from build123d import *

# Parameters (mm, degrees)
F0_W      = 50
F0_H      = 50
F1_DEPTH  = 12
F3_DEPTH  = 12
F5_W      = 7.196964696
F5_H      = 12
F6_DEPTH  = 25
F7_W      = 5.4
F7_H      = 5.4
F8_DEPTH  = 25
F9_W      = 5.4
F9_H      = 5.4
F9_W_2    = 4.6
F9_H_2    = 4.6
F10_DEPTH = 1
F11_R     = 0.19999
F13_W     = 25
F13_H     = 12
F14_DEPTH = 50
F15_W     = 25
F15_H     = 12
F16_DEPTH = 25
F17_COUNT = 4


# Not quite as in the source:
# - a fillet or chamfer that OpenCascade refuses, or shapes differently, is made with other operations: its cross-section is extruded or revolved along the edge and cut away or added
# - a fillet or chamfer is up to 0.001 mm smaller than in the source, because OpenCascade refuses the exact size


with BuildPart() as f1:
    # F0 (on Top) → F1 (new body)
    with BuildSketch(Plane.XY):
        Rectangle(F0_W, F0_H)
    extrude(amount=F1_DEPTH)

    # F2 (on face) → F3 (join)
    with BuildSketch(Plane(origin=(-25, 0, 0), x_dir=(0, -1, 0), z_dir=(-1, 0, 0))):
        with BuildLine():
            ThreePointArc((0, 0), (4.2426406871, 1.7573593129), (6, 6))
            ThreePointArc((6, 6), (4.2426406871, 10.2426406871), (0, 12))
            ThreePointArc((0, 12), (-6, 6), (0, 0))
        make_face()
    extrude(amount=F3_DEPTH)

    # F4: fillet of radius 6 on 1 edges, made by hand

    # F4_s1 → F4_t2 (revolve, cut)
    with BuildSketch(Plane.XZ):
        with BuildLine():
            ThreePointArc((-31, 12), (-35.2426406871, 10.2426406871), (-37, 6))
            Line((-37, 6), (-37.12, 6))
            Line((-37.12, 6), (-37.12, 12.12))
            Line((-37.12, 12.12), (-31, 12.12))
            Line((-31, 12.12), (-31, 12))
        make_face()
    revolve(axis=Axis((-37, 0, 6), (1, 0, 0)), mode=Mode.SUBTRACT)

    # F5 (on face) → F6 (cut)
    with BuildSketch(Plane(origin=(-25, 0, 0), x_dir=(0, -1, 0), z_dir=(-1, 0, 0))):
        with Locations((3.598482348, 6)):
            Rectangle(F5_W, F5_H)
    extrude(amount=F6_DEPTH, mode=Mode.SUBTRACT)

    # F7 (on face) → F8 (cut)
    with BuildSketch(Plane.XZ):
        with Locations((-31, 6)):
            Rectangle(F7_W, F7_H)
    extrude(amount=-F8_DEPTH, mode=Mode.SUBTRACT)

    # F9 (on face) → F10 (join)
    with BuildSketch(Plane.XZ):
        with Locations((-31, 6)):
            Rectangle(F9_W, F9_H)
        with Locations((-31, 6)):
            Rectangle(F9_W_2, F9_H_2, mode=Mode.SUBTRACT)
    extrude(amount=-F10_DEPTH)

    # F11 (radius 0.2 in the source; OpenCascade refuses exactly that, so slightly less here)
    f11_edges = [f1.edges().sort_by_distance(p)[0] for p in [
        (-28.7, 1, 6),
        (-28.3, 1, 6),
        (-31, 1, 8.7),
        (-31, 1, 8.3),
        (-33.7, 1, 6),
        (-33.3, 1, 6),
        (-31, 1, 3.3),
        (-31, 1, 3.7),
    ]]
    fillet(f11_edges, radius=F11_R)

    # F13 (on face) → F14 (cut)
    with BuildSketch(Plane(origin=(-25, 0, 0), x_dir=(0, -1, 0), z_dir=(-1, 0, 0))):
        with Locations((12.5, 6)):
            Rectangle(F13_W, F13_H)
    extrude(amount=-F14_DEPTH, mode=Mode.SUBTRACT)

    # F15 (on face) → F16 (cut)
    with BuildSketch(Plane(origin=(0, 25, 0), x_dir=(-1, 0, 0), z_dir=(0, 1, 0))):
        with Locations((-12.5, 6)):
            Rectangle(F15_W, F15_H)
    extrude(amount=-F16_DEPTH, mode=Mode.SUBTRACT)

    # F17: F1 ×4 about axis
    f17_axis = Axis((0, 0, 13.6458836496), (0, 0, 1))


with BuildPart() as f1_1:
    add(f1.part)
    for i in range(1, F17_COUNT):
        add(f1.part.rotate(f17_axis, i * 360 / F17_COUNT))


solid = f1_1.part
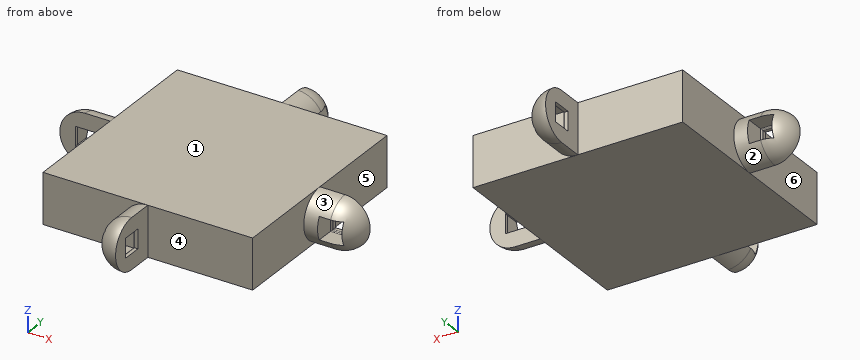
CAD build for the part. Positions are in the model's coordinates, mm. Face numbers are marked on the shaded views. A direction names the side the tool comes from. Give positions to 0.01 mm unless a question says otherwise; leave off trailing zeros. Order: outer loops, then holes, each group sorted by start corner. A loop starts at its lowest first (then second) coordinate and runs counter-clockwise, first axis right, second up. Notation, with made-up numbers: (-31.5, 66) - (-10.5, 66) arc R11 cw to (-10.5, 75) - close; hole circle Ø11 at (-11.75, 51.25). An arc over 180 degrees is marked (long way). Answer in a Markdown table with one row per item.
1. Saw through at D-D, the plane z = 1.75. Give the cut face in (x, y), plus the area to 3 significant figures.
Data:
| item | result |
|---|---|
| outline | (-35.24, 0) - (-25, 0) - (-25, -25) - (-4.24, -25) - (-4.24, -31) arc R4.24 ccw to (0, -35.24) - (0, -25) - (25, -25) - (25, -4.24) - (31, -4.24) arc R4.24 ccw to (35.24, 0) - (25, 0) - (25, 25) - (4.24, 25) - (4.24, 31) arc R4.24 ccw to (0, 35.24) - (0, 25) - (-25, 25) - (-25, 4.24) - (-31, 4.24) arc R4.24 ccw to start |
| area | 2,660 mm² |
2. Saw through at B-B, the plane y = -3.5. Give the cut face in (x, z).
Data:
| item | result |
|---|---|
| outline | (-25, 0) - (25, 0) - (25, 1.13) - (31, 1.13) arc R4.87 ccw to (31, 10.87) - (25, 10.87) - (25, 12) - (-25, 12) - close; hole (28.3, 3.3) - (33.7, 3.3) - (33.7, 8.7) - (28.3, 8.7) - close |
3. Probe probe 1 along X at (y, z) = (18, 4.5); probe 2 along X at (y, z) = (-3.5, 5.5). List the from-to ranges inside material, lowest first. Write a range as [from, to].
Data:
| item | result |
|---|---|
| probe 1 | x = [-25, 25] |
| probe 2 | x = [-25, 28.3], [33.7, 35.85] |
4. Tool access for the marked faces 4, 5 and 6: list every direction of +Z, -Z, +X, -X, +Y, -Y with a clear straight run to the whole face (end or side of a thin tool).
Data:
| item | result |
|---|---|
| face 4 | +Z, -Z, +X, -Y |
| face 5 | +Z, -Z, +X, +Y |
| face 6 | +Z, -Z, -X, -Y |
5. Saw through at A-A, the plane z = 6. Count the separate pieces of the cut face and the enclosed holes in it, plus the area to 3 significant figures.
Data:
| item | result |
|---|---|
| separate pieces | 5 |
| enclosed holes | 0 |
| area | 2,630 mm² |
6. Saw through at C-C, the plane x = 2.5. Give the cut face in (y, z), plus the area to 3 significant figures.
Data:
| item | result |
|---|---|
| outline | (-25, 0) - (25, 0) - (25, 0.55) - (31, 0.55) arc R5.45 ccw to (31, 11.45) - (25, 11.45) - (25, 12) - (-25, 12) - close; hole (28.3, 3.3) - (33.7, 3.3) - (33.7, 8.7) - (28.3, 8.7) - close |
| area | 683 mm² |
7. Pull direction Y, two halves, no side cores. Call the marked faces 1, 2 and 3: pulls with the +Y half, pulls with the -Y half, needs draft (parallel to the pull), parting line crosses it, or undercut.
Data:
| item | result |
|---|---|
| face 1 | needs draft |
| face 2 | pulls with the +Y half |
| face 3 | pulls with the -Y half |
8. Flat gauge pins, fed straight in: pin 1 (0.9 mm diameter, centred on x = -0.5, z = 7, fed in from +Y); pin 2 (1.5 mm diameter, centred on y = -30.5, z = 6.5, fed in from -X); pin 3 (6 mm diameter, centred on y = 11.5, z = 7, fed in from +X); pin 4 (4.5 mm diameter, centred on x = 4, y = 31, fed in from -Z). Where does each tip first touch, or does it go through?
Data:
| item | result |
|---|---|
| pin 1 | stops at y = 25 |
| pin 2 | passes through |
| pin 3 | stops at x = 25 |
| pin 4 | stops at z = 0.26 |
